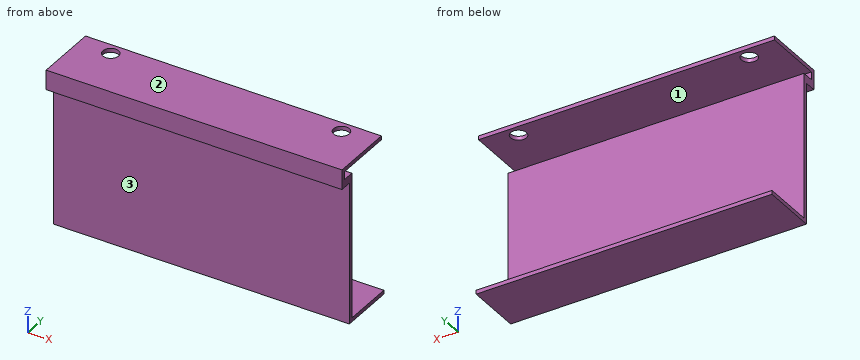
from build123d import *

# Parameters (mm, degrees)
ESQUISSE1_W             = 75
ESQUISSE1_H             = 15
ESQUISSE1_R             = 2
ESQUISSE1_H_2           = 1
BOSS_EXTRU_1_DEPTH      = 1
ESQUISSE1_3_W           = 75
ESQUISSE1_3_H           = 1
BOSS_EXTRU_2_DEPTH      = 40
ESQUISSE2_W             = 75
ESQUISSE2_H             = 1
BOSS_EXTRU_3_DEPTH      = 16
ESQUISSE3_W             = 65
ESQUISSE3_H             = 33
ENL_V_MAT_EXTRU_1_DEPTH = 3
ESQUISSE4_W             = 75
ESQUISSE4_H             = 37
BOSS_EXTRU_4_DEPTH      = 3
ESQUISSE5_W             = 75
ESQUISSE5_H             = 36
ENL_V_MAT_EXTRU_2_DEPTH = 3


with BuildPart() as part:
    # Esquisse1 → Boss.-Extru.1 (new body)
    # profile 1 of 2: a face of its own
    with BuildSketch(Plane.XY):
        with Locations((37.5, 7.5)):
            Rectangle(ESQUISSE1_W, ESQUISSE1_H)
        with Locations((66.75, 12)):
            Circle(ESQUISSE1_R, mode=Mode.SUBTRACT)
        with Locations((8.25, 12)):
            Circle(ESQUISSE1_R, mode=Mode.SUBTRACT)
    # profile 2 of 2: a face of its own
    with BuildSketch(Plane.XY):
        with Locations((37.5, -0.5)):
            Rectangle(ESQUISSE1_W, ESQUISSE1_H_2)
    extrude(amount=BOSS_EXTRU_1_DEPTH)

    # Esquisse1_3 → Boss.-Extru.2 (add)
    with BuildSketch(Plane.XY):
        with Locations((37.5, -0.5)):
            Rectangle(ESQUISSE1_3_W, ESQUISSE1_3_H)
    extrude(amount=-BOSS_EXTRU_2_DEPTH)

    # Esquisse2 → Boss.-Extru.3 (add)
    with BuildSketch(Plane(origin=(0, 0, 0), x_dir=(1, 0, 0), z_dir=(0, 1, 0))):
        with Locations((37.5, 39.5)):
            Rectangle(ESQUISSE2_W, ESQUISSE2_H)
    extrude(amount=BOSS_EXTRU_3_DEPTH)

    # Esquisse3 → Enl_v. mat.-Extru.1 (cut)
    with BuildSketch(Plane.XZ.offset(1)):
        with Locations((37.5, -20.5)):
            Rectangle(ESQUISSE3_W, ESQUISSE3_H)
    extrude(amount=-ENL_V_MAT_EXTRU_1_DEPTH, mode=Mode.SUBTRACT)

    # Esquisse4 → Boss.-Extru.4 (add)
    with BuildSketch(Plane(origin=(0, 0, 0), x_dir=(1, 0, 0), z_dir=(0, 1, 0))):
        with Locations((37.5, 20.5)):
            Rectangle(ESQUISSE4_W, ESQUISSE4_H)
    extrude(amount=BOSS_EXTRU_4_DEPTH)

    # Esquisse5 → Enl_v. mat.-Extru.2 (cut)
    with BuildSketch(Plane.XZ.offset(1)):
        with Locations((37.5, -22)):
            Rectangle(ESQUISSE5_W, ESQUISSE5_H)
    extrude(amount=-ENL_V_MAT_EXTRU_2_DEPTH, mode=Mode.SUBTRACT)


solid = part.part
Here's how the part is built. I have some questions about the finished solid (model axes, mm). Face numbers are marked on the shaded views. A direction names the side the tool comes from. Give positions to 0.01 mm unless a question says otherwise; leave off trailing zeros. Loops run counter-clockwise (first coordinate to the right, second up) from the corner with the lowest first, then second, coordinate; pieces in that order, holes last. Notation, with made-up numbers: (71, 12.5) -> (113, 12.5) arc R34 ccw to (113, 50.5) -> close; hole circle Ø1 at (32, -37.75). An arc over 180 degrees is marked (long way). Answer as a JSON object with one key per item and string values. Group by question number.
Item 1: Will these pins go through, and if not, where does the flat tip stop? pin 1 (4 mm diameter, centred on x = 30, z = -18, fed in from +Y); pin 2 (1.5 mm diameter, centred on x = 40.5, y = 0.5, fed in from -Z); pin 3 (12 mm diameter, centred on x = 57.5, z = -12.5, fed in from -Y); pin 4 (2 mm diameter, centred on x = 48, y = 1.5, fed in from -Z).
Item 2: Imagine slicing it at B-B on y = 12. Write out the boundary of the cut face in (x, z), then the cut area to 3 significant figures.
Item 3: Imagine slicing it at A-A on x = 66.75. Write out the boundary of the cut face in (y, z), then the cut area to 3 significant figures.
Item 4: Imagine slicing it at C-C on y = 7.25. Write out the boundary of the cut face in (x, z), then the cut area to 3 significant figures.
Item 5: On a 3-axis mill with a long thin cutter (end or side, diameter ignored), from which of +Z, -Z, +X, -X, +Y, -Y can I reach the whole of each face in a straight line? I mean the marked faces 1, 2 and 3. Say none if no direction works.
Item 6: Imagine slicing it at D-D on x = 21. Write out the boundary of the cut face in (y, z), then the cut area to 3 significant figures.
Item 7: I need wall thicknesses on L1, parallel to Z at x = 28.5, y = 13.25; L2, parallel to Z at x = 53, y = 0.25; L3, parallel to Y at x = 8.25, z = 0.7. Which ranges of each line are inside material? Lowest first, please.
Answer list:
{
 "1": {"pin 1": "stops at y = 3", "pin 2": "stops at z = -4", "pin 3": "stops at y = 2", "pin 4": "stops at z = -40"},
 "2": {"outline": "(0, -40) -> (75, -40) -> (75, -39) -> (0, -39) -> close; (0, 0) -> (6.25, 0) -> (6.25, 1) -> (0, 1) -> close; (10.25, 0) -> (64.75, 0) -> (64.75, 1) -> (10.25, 1) -> close; (68.75, 0) -> (75, 0) -> (75, 1) -> (68.75, 1) -> close", "area": "142 mm2"},
 "3": {"outline": "(-1, -4) -> (2, -4) -> (2, -40) -> (16, -40) -> (16, -39) -> (3, -39) -> (3, -2) -> (0, -2) -> (0, 0) -> (10, 0) -> (10, 1) -> (-1, 1) -> close; (14, 0) -> (15, 0) -> (15, 1) -> (14, 1) -> close", "area": "71.0 mm2"},
 "4": {"outline": "(0, -40) -> (75, -40) -> (75, -39) -> (0, -39) -> close; (0, 0) -> (75, 0) -> (75, 1) -> (0, 1) -> close", "area": "150 mm2"},
 "5": {"face 1": "+X, -X, +Y", "face 2": "+Z, +X, -X, +Y, -Y", "face 3": "-Z, +X, -X, -Y"},
 "6": {"outline": "(-1, -4) -> (2, -4) -> (2, -40) -> (16, -40) -> (16, -39) -> (3, -39) -> (3, -2) -> (0, -2) -> (0, 0) -> (15, 0) -> (15, 1) -> (-1, 1) -> close", "area": "75.0 mm2"},
 "7": {"L1": "z = -40 to -39, 0 to 1", "L2": "z = -4 to -2, 0 to 1", "L3": "y = -1 to 10, 14 to 15"}
}
